Model file for the job. Use its own axes, mm. A direction names the side the tool comes from. Round coordinates to 2 decimals unless told otherwise and drop trailing zeros. Order: outer loops, then holes, each group sorted by start corner. A loop starts at its lowest first (then second) coordinate and runs counter-clockwise, first axis right, second up. Notation, with made-up numbers: (-26, 7) - (9, 7) arc R15 cw to (9, 14) - close; hole circle Ø8 at (34.5, -0.75). An arc over 180 degrees is marked (long way). Put each result on its own line as item: value. Start each with the question number.
Item 1: Pin check, flat tips, straight feed: pin 1 Ø3 at (y, z) = (-7.5, 14.5) entering from +X; pin 2 Ø2 at (y, z) = (-19.17, 7.94) entering from +X; pin 3 Ø1.5 at (x, z) = (3.5, -15.5) entering from +Y; pin 4 Ø1.1 at (x, z) = (4, -18.5) entering from -Y. Stop position of each tip, or through.
Item 2: Saw through at B-B on y = 6. List the corners of the cut face in (x, z).
Item 3: Saw through at A-A on z = 0. List the corners of the cut face in (x, y).
Item 4: Saw through at C-C on x = 4. State how many separate pieces and enclosed holes the cut face has, plus the area to 3 significant figures.
Item 5: Mould opens along Y. For faces 4 (the face through (4, -35.29, 19)), 5 (the face through (0, -15, 5)), 6 (the face through (3.944, -8.419, 18.016)) say: pulls with the +Y half, pulls with the -Y half, needs draft (parallel to the pull), parting line crosses it, or undercut.
Item 6: Which spindle directions (+Z, -Z, +X, -X, +Y, -Y) get a long thin tool onto all of the face, cutting with end or side? Do faces 1 (the face through (4.541, -37.825, -17.283)), 2 (the face through (5, -11.4, 14.8)), 3 (the face through (4, -20, 23)). Say none if no direction does.
Item 7: Probe probe 1 along Z at (x, y) = (0.5, -19); probe 2 along Y at (x, z) = (0.75, -8); probe 3 along Z at (x, y) = (6, 20). List the from-to ranges inside material, lowest first.
```python
from build123d import *

# Parameters (mm, degrees)
SKETCH_1_R          = 18.68
SKETCH_1_R_2        = 15.652173913
EXTRUDE_2_DEPTH     = 2
SKETCH_1_4_R        = 23
SKETCH_1_4_R_2      = 1.25
SKETCH_1_4_R_3      = 18.68
EXTRUDE_3_DEPTH     = 8
EXTRUDE_4_DEPTH     = 8
SKETCH_3_R          = 1.8
CUT_EXTRUDE_1_DEPTH = 5


with BuildPart() as part:
    # Sketch 1 → Extrude 2 (new body)
    with BuildSketch(Plane(origin=(0, 0, 0), x_dir=(0, 0, -1), z_dir=(1, 0, 0))):
        Circle(SKETCH_1_R)
        Circle(SKETCH_1_R_2, mode=Mode.SUBTRACT)
    extrude(amount=EXTRUDE_2_DEPTH)

    # Sketch 1_4 → Extrude 3 (add)
    with BuildSketch(Plane(origin=(0, 0, 0), x_dir=(0, 0, -1), z_dir=(1, 0, 0))):
        Circle(SKETCH_1_4_R)
        with Locations((-7.940681222, 19.1705003)):
            Circle(SKETCH_1_4_R_2, mode=Mode.SUBTRACT)
        with Locations((-19.1705003, 7.940681222)):
            Circle(SKETCH_1_4_R_2, mode=Mode.SUBTRACT)
        with Locations((-19.1705003, -7.940681222)):
            Circle(SKETCH_1_4_R_2, mode=Mode.SUBTRACT)
        with Locations((-7.940681222, -19.1705003)):
            Circle(SKETCH_1_4_R_2, mode=Mode.SUBTRACT)
        with Locations((7.940681222, -19.1705003)):
            Circle(SKETCH_1_4_R_2, mode=Mode.SUBTRACT)
        with Locations((19.1705003, -7.940681222)):
            Circle(SKETCH_1_4_R_2, mode=Mode.SUBTRACT)
        with Locations((19.1705003, 7.940681222)):
            Circle(SKETCH_1_4_R_2, mode=Mode.SUBTRACT)
        with Locations((7.940681222, 19.1705003)):
            Circle(SKETCH_1_4_R_2, mode=Mode.SUBTRACT)
        Circle(SKETCH_1_4_R_3, mode=Mode.SUBTRACT)
    extrude(amount=EXTRUDE_3_DEPTH)

    # Sketch 2 → Extrude 4 (add)
    with BuildSketch(Plane.ZY):
        with BuildLine():
            Line((-23, -40.29), (-23, 0))
            ThreePointArc((-23, 0), (0, -23), (23, 0))
            Line((23, 0), (23, -40.29))
            Line((23, -40.29), (-23, -40.29))
        make_face()
    extrude(amount=-EXTRUDE_4_DEPTH)

    # Sketch 3 → Cut-Extrude 1 (cut)
    with BuildSketch(Plane.XZ.offset(40.29)):
        with Locations(Location((4, 19, 0), (0, 0, 270))):
            Circle(SKETCH_3_R)
    cut_extrude_1 = extrude(amount=-CUT_EXTRUDE_1_DEPTH, mode=Mode.SUBTRACT)

    # Mirror 1: Cut-Extrude 1 across plane
    add(cut_extrude_1.mirror(Plane(origin=(0, 0, 0), x_dir=(1, 0, 0), z_dir=(0, 0, -1))), mode=Mode.SUBTRACT)


solid = part.part
```
Results found:
1. pin 1: stops at x = 2
1. pin 2: passes through
1. pin 3: stops at y = 17.65
1. pin 4: stops at y = -35.29
2. outline: (0, -22.2) - (8, -22.2) - (8, -17.69) - (2, -17.69) - (2, -14.46) - (0, -14.46) - close; (0, 14.46) - (2, 14.46) - (2, 17.69) - (8, 17.69) - (8, 22.2) - (0, 22.2) - close
3. outline: (0, -40.29) - (8, -40.29) - (8, -18.68) - (2, -18.68) - (2, -15.65) - (0, -15.65) - close; (0, 15.65) - (2, 15.65) - (2, 18.68) - (8, 18.68) - (8, 23) - (0, 23) - close
4. separate pieces: 1
4. enclosed holes: 9
4. area: 1,510 mm²
5. face 4: pulls with the -Y half
5. face 5: needs draft
5. face 6: undercut
6. face 1: -Y
6. face 2: +X
6. face 3: +Z, +X, -X, +Y, -Y
7. probe 1: z = -23 to -9.18, -6.7 to 6.7, 9.18 to 23
7. probe 2: y = -40.29 to -20.42, -17.92 to -13.45, 13.45 to 17.92, 20.42 to 21.56
7. probe 3: z = -11.36 to -8.88, -7.01 to 7.01, 8.88 to 11.36
